from build123d import *

# Parameters (mm, degrees)
BOSS_EXTRUDE1_DEPTH = 7
CUT_EXTRUDE1_DEPTH  = 5
FILLET1_R           = 1
SKETCH3_R           = 1
CUT_EXTRUDE2_DEPTH  = 14.304134756


with BuildPart() as part:
    # Sketch1 → Boss-Extrude1 (new, symmetric)
    with BuildSketch(Plane.XY):
        with BuildLine():
            Line((-8, 0), (-4, 0))
            ThreePointArc((-4, 0), (0, 4), (4, 0))
            Line((4, 0), (8, 0))
            ThreePointArc((8, 0), (0, 8), (-8, 0))
        make_face()
    extrude(amount=BOSS_EXTRUDE1_DEPTH, both=True)

    # Sketch2 → Cut-Extrude1 (cut, symmetric)
    with BuildSketch(Plane.XY):
        with BuildLine():
            Line((-8, 0), (-6, 0))
            ThreePointArc((-6, 0), (0, 6), (6, 0))
            Line((6, 0), (8, 0))
            ThreePointArc((8, 0), (0, 8), (-8, 0))
        make_face()
    extrude(amount=CUT_EXTRUDE1_DEPTH, both=True, mode=Mode.SUBTRACT)

    # Fillet1
    fillet1_edges = [part.edges().sort_by_distance(p)[0] for p in [
        (0, 8, 7),
        (0, 8, -7),
    ]]
    fillet(fillet1_edges, radius=FILLET1_R)

    # Sketch3 → Cut-Extrude2 (cut, through all)
    with BuildSketch(Plane(origin=(0, 0, 0), x_dir=(1, 0, 0), z_dir=(0, 1, 0))):
        with Locations(Location((0, 0, 0), (0, 0, 90))):
            Circle(SKETCH3_R)
    extrude(amount=CUT_EXTRUDE2_DEPTH, mode=Mode.SUBTRACT)


solid = part.part
Could you check a few things on this model? Use its own coordinates, in mm. A direction names the side the tool comes from. Give positions to 0.01 mm unless a question says otherwise; leave off trailing zeros. Order: outer loops, then holes, each group sorted by start corner. A loop starts at its lowest first (then second) coordinate and runs counter-clockwise, first axis right, second up. Notation, with made-up numbers: (54, 86) - (109, 86) arc R8 cw to (109, 98) - close; hole circle Ø4 at (22.25, 13). An arc over 180 degrees is marked (long way). One line per item, written item: value. Start each with the question number.
1. Imagine slicing it at B-B on z = 0. List the corners of the cut face in (x, y) for me.
2. For P1, Ø3, axis at x = 1, z = -0.5, coming from the +Y side; P2, Ø1.5, axis at x = -2.5, z = -4.5, coming from the +Y side; P3, Ø5, axis at x = -0.5, z = 0.5, coming from the -Y side, each with a flat end and sliding along its axis, tell me the tip position at first contact or that it passes through.
3. Thinking about a two-plate mould opening in Z: for faces 1 (the face through (-5, 0, 0)), 2 (the face through (-0.1, 4.3, 7)), 3 (the face through (0, 5, 1)), which applies, +Z half, -Z half, draft (parallel to the pull), parting line (faces both ways), or undercut?
4. Imagine slicing it at A-A on x = 0. List the corners of the cut face in (y, z) for me, plus the area to 3 significant figures.
5. Imagine slicing it at D-D on z = -5.25. List the corners of the cut face in (x, y) for me.
6. Imagine slicing it at C-C on z = -3.75. List the corners of the cut face in (x, y) for me.
7. If I drill on probe 1 along Z at (x, y) = (4, 5.5); probe 2 along X at (y, z) = (1.25, -0.5); probe 3 along X at (y, z) = (5.45, 0), over which ranges is the centre line in solid material (lowest first)?
8. For faces 4 (the face through (0, 7, -5)), 5 (the face through (-0.1, 4.3, -7)), which set-ups out of +Z, -Z, +X, -X, +Y, -Y let a thin tool reach every point of the face, with its end or its side?
Values:
1. outline: (-6, 0) - (-4, 0) arc R4 cw to (-1, 3.87) - (-1, 5.92) arc R6 ccw to start; (1, 3.87) arc R4 cw to (4, 0) - (6, 0) arc R6 ccw to (1, 5.92) - close
2. P1: y = 6
2. P2: y = 7.76
2. P3: y = 2.65
3. face 1: draft
3. face 2: +Z half
3. face 3: undercut
4. outline: (4, -7) - (7, -7) arc R1 ccw to (8, -6) - (8, -5) - (6, -5) - (6, -1) - (4, -1) - close; (4, 1) - (6, 1) - (6, 5) - (8, 5) - (8, 6) arc R1 ccw to (7, 7) - (4, 7) - close
4. area: 31.6 mm²
5. outline: (-8, 0) - (-4, 0) arc R4 cw to (4, 0) - (8, 0) arc R8 ccw to start
6. outline: (-6, 0) - (-4, 0) arc R4 cw to (4, 0) - (6, 0) arc R6 ccw to start
7. probe 1: -7 to -5, 5 to 7
7. probe 2: -5.87 to -3.8, 3.8 to 5.87
7. probe 3: -2.51 to -1, 1 to 2.51
8. face 4: +Y
8. face 5: -Z, +X, -X, +Y, -Y
